Could you check a few things on this drawing? It's one solid part, dimensions in mm from its lowest x, y, z. A direction names the side the tool comes from. Coordinates: 2 decimals unless noted, no trailing zeros. Loops run counter-clockwise (first coordinate to the right, second up) from the corner with the lowest first, then second, coordinate; pieces in that order, holes last.
1) Will these pins go through, and if not, where does the flat tip stop? P1, Ø5, axis at y = 6.5, z = 21.5, coming from the -X side; P2, Ø2, axis at x = 26.5, z = 60, coming from the -Y side; P3, Ø10, axis at x = 27, y = 11.5, coming from the +Z side.
2) Imagine slicing it at A-A on z = 47. Please give me the cut outline in (x, y), plus the area to 3 significant figures.
3) Imagine slicing it at B-B on x = 51.5. Please give me the cut outline in (y, z), plus the area to 3 significant figures.
4) If I drill on line 1 along X through (y, z) = (5, 77.5); line 2 along Z through (x, y) = (30.5, 19.25); line 3 along X through (y, z) = (19.25, 10), over which ranges is the centre line in solid material (lowest first)?
5) Imagine slicing it at D-D on z = 90. Please give me the cut outline in (x, y), plus the area to 3 significant figures.
6) For the marked faces 1, 2, 3 and 4, which set-ups out of +Z, -Z, +X, -X, +Y, -Y let a thin tool reach every point of the face, with its end or its side?
7) Imagine slicing it at C-C on y = 15.5. Please give me the cut outline in (x, z).
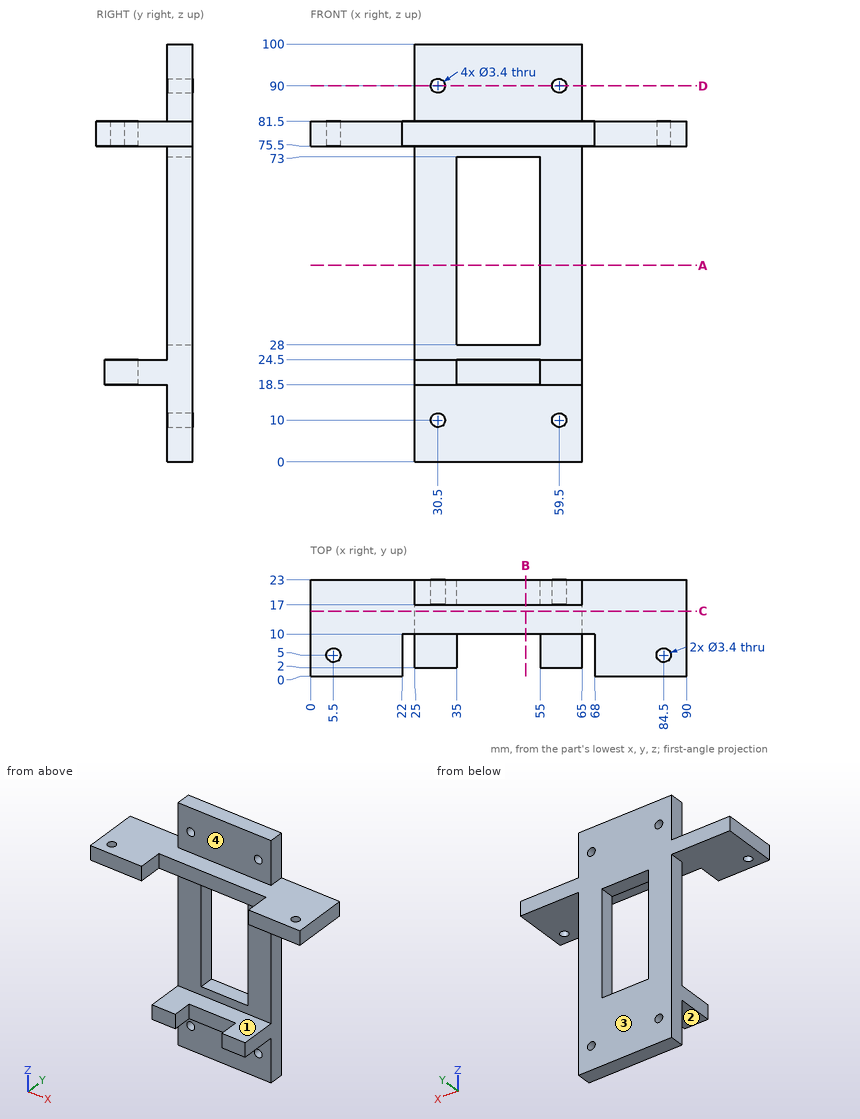
Filled in:
1. P1: stops at x = 25
1. P2: stops at y = 17
1. P3: stops at z = 81.5
2. outline: (25, 17) - (35, 17) - (35, 23) - (25, 23) - close; (55, 17) - (65, 17) - (65, 23) - (55, 23) - close
2. area: 120 mm2
3. outline: (10, 18.5) - (17, 18.5) - (17, 0) - (23, 0) - (23, 28) - (17, 28) - (17, 24.5) - (10, 24.5) - close; (10, 75.5) - (17, 75.5) - (17, 73) - (23, 73) - (23, 100) - (17, 100) - (17, 81.5) - (10, 81.5) - close
3. area: 414 mm2
4. line 1: x = 0 to 3.8, 7.2 to 22, 68 to 82.8, 86.2 to 90
4. line 2: z = 0 to 8.3, 11.7 to 88.3, 91.7 to 100
4. line 3: x = 25 to 28.8, 32.2 to 57.8, 61.2 to 65
5. outline: (25, 17) - (28.8, 17) - (28.8, 23) - (25, 23) - close; (32.2, 17) - (57.8, 17) - (57.8, 23) - (32.2, 23) - close; (61.2, 17) - (65, 17) - (65, 23) - (61.2, 23) - close
5. area: 199 mm2
6. face 1: +X, -X, -Y
6. face 2: -Z, +X, -X, -Y
6. face 3: +Z, -Z, +X, -X, +Y
6. face 4: +Z, +X, -X, -Y
7. outline: (0, 75.5) - (90, 75.5) - (90, 81.5) - (0, 81.5) - close; (25, 18.5) - (65, 18.5) - (65, 24.5) - (25, 24.5) - close
